Here's how the part is built. I have some questions about the finished solid (model axes, mm). A direction names the side the tool comes from. Round coordinates to 2 decimals unless told otherwise and drop trailing zeros. Loops run counter-clockwise (first coordinate to the right, second up) from the corner with the lowest first, then second, coordinate; pieces in that order, holes last. Notation, with made-up numbers: M 36,63 L 73,63 A28 cw 73,91 Z; hole C 8.25,82 d4. An arc over 180 degrees is marked long. Answer as a JSON object with one key per item and string values.
from build123d import *

# Parameters (mm, degrees)
F2_R     = 17.975364
F3_DEPTH = 130
F4_R     = 5
F5_R     = 5


with BuildPart() as f1:
    # F0 (on Front) → F1 (revolve)
    with BuildSketch(Plane.XZ):
        with BuildLine():
            Line((0, -50), (0, 50))
            ThreePointArc((0, 50), (-50, 0), (0, -50))
        make_face()
    revolve(axis=Axis((0, 0, 0), (0, 0, -1)))

    # F2 (on Top) → F3 (join)
    with BuildSketch(Plane.XY):
        Circle(F2_R)
    extrude(amount=F3_DEPTH)

    # F4
    f4_edges = [f1.edges().sort_by_distance(p)[0] for p in [
        (0, -17.975364, 46.657114),
        (0, 17.975364, 46.657114),
    ]]
    fillet(f4_edges, radius=F4_R)

    # F5
    f5_edges = [f1.edges().sort_by_distance(p)[0] for p in [
        (-17.975364, 0, 130),
    ]]
    fillet(f5_edges, radius=F5_R)


solid = f1.part
Item 1: I want a section at A-A, the plane z = 82.5. Please give me the cut outline in (x, y).
Resolved:
{"outline": "C 0,0 d35.95"}
Item 2: Please list where these lines run through material, in increasing order: probe 1 along Z at (x, y) = (28, 34); probe 2 along Z at (x, y) = (26.5, 29.5); probe 3 along X at (y, z) = (-23.5, -26). Write a range as from..to.
Resolved:
{"probe 1": "-23.66..23.66", "probe 2": "-30.45..30.45", "probe 3": "-35.66..35.66"}
Item 3: I'm going to push flat-ended pins straight in: pin 1 Ø5 at (x, z) = (-5, 99) entering from -Y; pin 2 Ø3 at (x, y) = (-23.5, -27.5) entering from -Z; pin 3 Ø3 at (x, z) = (30.5, 16) entering from +Y. Where does each tip first touch, or does it pass through?
Resolved:
{"pin 1": "y = -17.8", "pin 2": "z = -36.02", "pin 3": "y = 37.61"}
Item 4: On a 3-axis mill with a long thin cutter (end or side, diameter ignored), from which of +Z, -Z, +X, -X, +Y, -Y can I reach the whole of each face in a straight line? I mean faces 1 (the face through (0, 0, 130)), 2 (the face through (17.145, 5.399, 86.96)). Say none if no direction works.
Resolved:
{"face 1": "+Z, +X, -X, +Y, -Y", "face 2": "+Z"}
Item 5: I want a section at B-B, the plane x = -24. Please give me the cut outline in (y, z).
Resolved:
{"outline": "C 0,0 d87.73"}
